from build123d import *

# Parameters (mm, degrees)
SKETCH1_R           = 10
SKETCH1_R_2         = 8.985
BOSS_EXTRUDE1_DEPTH = 0.7
SKETCH2_R           = 10
SKETCH2_R_2         = 6
BOSS_EXTRUDE2_DEPTH = 7
SKETCH3_R           = 10
BOSS_EXTRUDE3_DEPTH = 1
SKETCH4_R           = 10
BOSS_EXTRUDE4_DEPTH = 2.5


with BuildPart() as part:
    # Sketch1 → Boss-Extrude1 (new body)
    with BuildSketch(Plane(origin=(0, 0, 0), x_dir=(1, 0, 0), z_dir=(0, 1, 0))):
        with Locations(Location((0, 0, 0), (0, 0, 270))):
            Circle(SKETCH1_R)
        with Locations(Location((0, 0, 0), (0, 0, 270))):
            Circle(SKETCH1_R_2, mode=Mode.SUBTRACT)
    extrude(amount=BOSS_EXTRUDE1_DEPTH)

    # Sketch2 → Boss-Extrude2 (add)
    with BuildSketch(Plane(origin=(0, 0.7, 0), x_dir=(1, 0, 0), z_dir=(0, 1, 0))):
        with Locations(Location((0, 0, 0), (0, 0, 270))):
            Circle(SKETCH2_R)
        with Locations(Location((0, 0, 0), (0, 0, 270))):
            Circle(SKETCH2_R_2, mode=Mode.SUBTRACT)
    extrude(amount=BOSS_EXTRUDE2_DEPTH)

    # Sketch3 → Boss-Extrude3 (add)
    with BuildSketch(Plane(origin=(0, 7.7, 0), x_dir=(1, 0, 0), z_dir=(0, 1, 0))):
        with Locations(Location((0, 0, 0), (0, 0, 270))):
            Circle(SKETCH3_R)
    extrude(amount=BOSS_EXTRUDE3_DEPTH)

    # Sketch4 → Boss-Extrude4 (add)
    with BuildSketch(Plane(origin=(0, 8.7, 0), x_dir=(1, 0, 0), z_dir=(0, 1, 0))):
        with Locations(Location((0, 0, 0), (0, 0, 270))):
            Circle(SKETCH4_R)
        with BuildLine():
            Line((-0.98, 2.98), (0.98, 2.98))
            ThreePointArc((0.98, 2.98), (2.394213562, 2.394213562), (2.98, 0.98))
            Line((2.98, 0.98), (2.98, -0.98))
            ThreePointArc((2.98, -0.98), (2.394213562, -2.394213562), (0.98, -2.98))
            Line((0.98, -2.98), (-0.98, -2.98))
            ThreePointArc((-0.98, -2.98), (-2.394213562, -2.394213562), (-2.98, -0.98))
            Line((-2.98, -0.98), (-2.98, 0.98))
            ThreePointArc((-2.98, 0.98), (-2.394213562, 2.394213562), (-0.98, 2.98))
        make_face(mode=Mode.SUBTRACT)
    extrude(amount=BOSS_EXTRUDE4_DEPTH)


solid = part.part
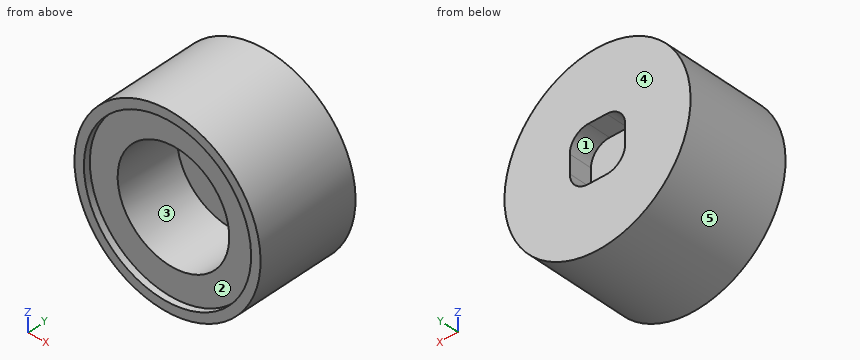
Can you work these out from the model? Positions are in its coordinate system, mm. Face numbers are marked on the shaded views. A direction names the side the tool comes from. Round coordinates to 2 decimals unless told otherwise and drop trailing zeros. Write each loop counter-clockwise with the first axis right and the second up, starting at its lowest first coordinate (ties: lowest second). Pieces come first, ordered by that corner, then holes. Notation, with made-up numbers: M -5.5,84.5 L 16.5,84.5 A26 ccw 16.5,104.5 Z; hole C -37,63.25 d11. An arc over 180 degrees is marked long. Use a Markdown table: item, result.
Item 1: For pin 1 Ø1.5 at (x, y) = (-8, 8) entering from -Z; pin 2 Ø1 at (x, z) = (-6.5, 4) entering from -Y; pin 3 Ø4 at (x, y) = (3.5, 5) entering from +Z, each with a flat end and sliding along its axis, tell me the tip position at first contact or that it passes through.
Found:
| item | result |
|---|---|
| pin 1 | stops at z = -6.89 |
| pin 2 | stops at y = 0.7 |
| pin 3 | stops at z = 9.89 |
Item 2: We'd pull the mould along Z, two halves only. Please class the marked faces 3, 4 and 5: released by +Z, released by -Z, zero draft, split by the parting line, or undercut.
Found:
| item | result |
|---|---|
| face 3 | undercut |
| face 4 | zero draft |
| face 5 | split by the parting line |
Item 3: I want a section at B-B (y = 10.5). List the corners of the cut face in (x, z) for me, and give its area (3 significant figures).
Found:
| item | result |
|---|---|
| outline | C 0,0 d20; hole M -2.98,-0.98 A2 ccw -0.98,-2.98 L 0.98,-2.98 A2 ccw 2.98,-0.98 L 2.98,0.98 A2 ccw 0.98,2.98 L -0.98,2.98 A2 ccw -2.98,0.98 Z |
| area | 282 mm2 |
Item 4: I want a section at C-C (x = -2). List the corners of the cut face in (y, z) for me.
Found:
| item | result |
|---|---|
| outline | M 0,-9.8 L 11.2,-9.8 L 11.2,-2.7 L 8.7,-2.7 L 8.7,2.7 L 11.2,2.7 L 11.2,9.8 L 0,9.8 L 0,8.76 L 0.7,8.76 L 0.7,5.66 L 7.7,5.66 L 7.7,-5.66 L 0.7,-5.66 L 0.7,-8.76 L 0,-8.76 Z |
Item 5: I want a section at D-D (x = 5.5). List the corners of the cut face in (y, z) for me.
Found:
| item | result |
|---|---|
| outline | M 0,-8.35 L 11.2,-8.35 L 11.2,8.35 L 0,8.35 L 0,7.1 L 0.7,7.1 L 0.7,2.4 L 7.7,2.4 L 7.7,-2.4 L 0.7,-2.4 L 0.7,-7.1 L 0,-7.1 Z |
Item 6: I want a section at A-A (z = 0). List the corners of the cut face in (x, y) for me (3 decimals).
Found:
| item | result |
|---|---|
| outline | M -10,0 L -8.985,0 L -8.985,0.7 L -6,0.7 L -6,7.7 L 6,7.7 L 6,0.7 L 8.985,0.7 L 8.985,0 L 10,0 L 10,11.2 L 2.98,11.2 L 2.98,8.7 L -2.98,8.7 L -2.98,11.2 L -10,11.2 Z |
Item 7: Which directions (+Z, -Z, +X, -X, +Y, -Y) give clear straight access to the entire face, cutting with the end or side of a thin tool? Please do the marked faces 1 and 2.
Found:
| item | result |
|---|---|
| face 1 | +Y |
| face 2 | -Y |
Item 8: If I drill on line 1 along X through (y, z) = (2.5, 0); line 2 along X through (y, z) = (0.55, 0) (3 decimals); line 3 along Y through (x, z) = (-0.5, 4.5), over which ranges is the centre line in solid material (lowest first)? Write a range as [from, to].
Found:
| item | result |
|---|---|
| line 1 | x = [-10, -6], [6, 10] |
| line 2 | x = [-10, -8.985], [8.985, 10] |
| line 3 | y = [7.7, 11.2] |
